from build123d import *

# Parameters (mm, degrees)
F0_R     = 4
F1_DEPTH = 15
F3_DEPTH = 5
F4_R     = 2
F5_DEPTH = 24.001
F6_R     = 10
F7_SIZE  = 1


with BuildPart() as f1:
    # F0 (on Top) → F1 (new body)
    with BuildSketch(Plane.XY):
        with BuildLine():
            Line((-30, -9), (-12, -9))
            ThreePointArc((-12, -9), (0, -15), (12, -9))
            Line((12, -9), (30, -9))
            Line((30, -9), (30, -2.5))
            Line((30, -2.5), (13, -2.5))
            Line((13, -2.5), (13, 0))
            Line((13, 0), (13, 2.5))
            Line((13, 2.5), (30, 2.5))
            Line((30, 2.5), (30, 9))
            Line((30, 9), (12, 9))
            ThreePointArc((12, 9), (0, 15), (-12, 9))
            Line((-12, 9), (-30, 9))
            Line((-30, 9), (-30, 2.5))
            Line((-30, 2.5), (-13, 2.5))
            Line((-13, 2.5), (-13, 0))
            Line((-13, 0), (-13, -2.5))
            Line((-13, -2.5), (-30, -2.5))
            Line((-30, -2.5), (-30, -9))
        make_face()
        Circle(F0_R, mode=Mode.SUBTRACT)
    extrude(amount=F1_DEPTH)

    # F2 (on face) → F3 (cut)
    with BuildSketch(Plane(origin=(0, 0, 0), x_dir=(1, 0, 0), z_dir=(0, 0, -1))):
        Polygon((3.752777, -6.5), (7.505553, 0), (3.752777, 6.5), (-3.752777, 6.5), (-7.505553, 0), (-3.752777, -6.5), align=None)
    extrude(amount=-F3_DEPTH, mode=Mode.SUBTRACT)

    # F4 (on face) → F5 (cut, through all)
    with BuildSketch(Plane.XZ.offset(9)):
        with Locations((-21, 10)):
            Circle(F4_R)
        with Locations((21, 10)):
            Circle(F4_R)
    extrude(amount=-F5_DEPTH, mode=Mode.SUBTRACT)

    # F6
    f6_edges = [f1.edges().sort_by_distance(p)[0] for p in [
        (-30, -5.75, 0),
        (-30, 5.75, 0),
        (30, -5.75, 0),
        (30, 5.75, 0),
    ]]
    fillet(f6_edges, radius=F6_R)

    # F7
    f7_edges = [f1.edges().sort_by_distance(p)[0] for p in [
        (-30, 5.75, 15),
        (-30, -5.75, 15),
        (30, 5.75, 15),
        (30, -5.75, 15),
    ]]
    chamfer(f7_edges, length=F7_SIZE)


solid = f1.part
Design review of the part built by this model. Coordinates are the model's own, in mm. A direction names the side the tool comes from. Coordinates: 2 decimals unless noted, no trailing zeros. Write each loop counter-clockwise with the first axis right and the second up, starting at its lowest first coordinate (ties: lowest second). Pieces come first, ordered by that corner, then holes. Notation, with made-up numbers: (-18.75, -38.5) - (3.25, -38.5) arc R16 ccw to (3.25, -27.5) - close; hole circle Ø10 at (67, -35). An arc over 180 degrees is marked (long way). Use one line per item in the form item = value.
Q1. Consider section C-C (z = 7.25). Write out the cut boundary in (x, y).
Taken from the geometry:
outline = (-29.61, -9) - (-12, -9) arc R15 ccw to (12, -9) - (29.61, -9) - (29.61, -2.5) - (13, -2.5) - (13, 2.5) - (29.61, 2.5) - (29.61, 9) - (12, 9) arc R15 ccw to (-12, 9) - (-29.61, 9) - (-29.61, 2.5) - (-13, 2.5) - (-13, -2.5) - (-29.61, -2.5) - close; hole circle Ø8 at (0, 0)
Q2. Consider section A-A (x = -25). Write out the cut boundary in (y, z), plus the area to 3 significant figures.
Taken from the geometry:
outline = (-9, 1.34) - (-2.5, 1.34) - (-2.5, 15) - (-9, 15) - close; (2.5, 1.34) - (9, 1.34) - (9, 15) - (2.5, 15) - close
area = 178 mm^2
Q3. Machinability: for faces 4 (the flat face through (21, 2.5, 7)), 5 (the flat face through (-21, 9, 7)), 6 (the flat face through (-21, -9, 7)), which of the approach directions +Z, -Z, +X, -X, +Y, -Y give a long, thin tool a straight path to every point of the face, cutting with its end or side? Answer none if there is none.
Taken from the geometry:
face_4 = +Z, -Z, +X
face_5 = +Z, -Z, -X, +Y
face_6 = +Z, -Z, -X, -Y
Q4. Consider section B-B (x = 21). Write out the cut boundary in (y, z), plus the area to 3 significant figures.
Taken from the geometry:
outline = (-9, 0.05) - (-2.5, 0.05) - (-2.5, 8) - (-9, 8) - close; (-9, 12) - (-2.5, 12) - (-2.5, 15) - (-9, 15) - close; (2.5, 0.05) - (9, 0.05) - (9, 8) - (2.5, 8) - close; (2.5, 12) - (9, 12) - (9, 15) - (2.5, 15) - close
area = 142 mm^2
Q5. The part is to be moulded in two halves that separate along X. For faces 1 (the flat face through (5.6, 3.3, 2.5)), 2 (the flat face through (13, 0, 7)), 3 (the flat face through (-21, -2.5, 7)), say which applies: +X half, -X half, draft (parallel to the pull), parting line (faces both ways), or undercut.
Taken from the geometry:
face_1 = undercut
face_2 = +X half
face_3 = draft
Q6. Insertion check: pin 1 Ø4 at (y, z) = (0, 7) entering from +X; pin 2 Ø3 at (y, z) = (8, 2.5) entering from +X; pin 3 Ø3 at (x, z) = (21, 10) entering from +Y; pin 4 Ø7.5 at (x, z) = (21.5, 4.5) entering from +Y. Each pin has a flat end and moves straight along its axis. Give the tip position at first contact, or say it passes through.
Taken from the geometry:
pin_1 = 13
pin_2 = 28
pin_3 = through
pin_4 = 9
Q7. Consider section D-D (x = 5). Write out the cut boundary in (y, z), plus the area to 3 significant figures.
Taken from the geometry:
outline = (-14.14, 0) - (-4.34, 0) - (-4.34, 5) - (4.34, 5) - (4.34, 0) - (14.14, 0) - (14.14, 15) - (-14.14, 15) - close
area = 381 mm^2
Q8. For probe 1 along Y at (x, z) = (26, 8.75); probe 2 along Z at (x, y) = (-21.5, 7.25); probe 3 along Z at (x, y) = (21, -4.25), list the stretches that pass through material, from the lowest coordinate up.
Taken from the geometry:
probe_1 = -9 to -2.5, 2.5 to 9
probe_2 = 0.11 to 8.06, 11.94 to 15
probe_3 = 0.05 to 8, 12 to 15
